from build123d import *

# Parameters (mm, degrees)
BOSS_EXTRUDE1_DEPTH = 25
FILLET1_R           = 70
FILLET2_R           = 5
CHAMFER1_SIZE       = 1
SKETCH2_R           = 2.25
CUT_EXTRUDE1_DEPTH  = 163.385344166
SKETCH5_W           = 8
SKETCH5_H           = 7
CUT_EXTRUDE2_DEPTH  = 322.199315068
CHAMFER2_SIZE       = 1


with BuildPart() as part:
    # Sketch1 → Boss-Extrude1 (new body)
    with BuildSketch(Plane(origin=(0, 0, 0), x_dir=(0, 0, -1), z_dir=(1, 0, 0))):
        Polygon((-160, 0), (160, 0), (160, -5), (100, -12), (-100, -12), (-160, -5), align=None)
    extrude(amount=BOSS_EXTRUDE1_DEPTH)

    # Fillet1
    fillet1_edges = [part.edges().sort_by_distance(p)[0] for p in [
        (12.5, -12, -100),
        (12.5, -12, 100),
    ]]
    fillet(fillet1_edges, radius=FILLET1_R)

    # Fillet2
    fillet2_edges = [part.edges().sort_by_distance(p)[0] for p in [
        (12.5, -5, -160),
        (12.5, -5, 160),
    ]]
    fillet(fillet2_edges, radius=FILLET2_R)

    # Chamfer1
    chamfer1_edges = [part.edges().sort_by_distance(p)[0] for p in [
        (25, -0.274710282, 160),
        (0, -8.522077997, -129.810760023),
        (25, -8.522077997, -129.810760023),
        (0, -12, 0),
        (0, -11.882005486, 99.99314025),
        (0, -11.882005486, -99.99314025),
        (25, -12, 0),
        (25, -11.882005486, 99.99314025),
        (25, -11.882005486, -99.99314025),
        (0, -0.274710282, -160),
        (25, -0.274710282, -160),
        (0, -8.522077997, 129.810760023),
        (0, -3.873798889, 158.73477024),
        (0, -3.873798889, -158.73477024),
        (25, -8.522077997, 129.810760023),
        (25, -3.873798889, 158.73477024),
        (25, -3.873798889, -158.73477024),
        (0, -0.274710282, 160),
    ]]
    chamfer(chamfer1_edges, length=CHAMFER1_SIZE)

    # Sketch2 → Cut-Extrude1 (cut, through all)
    with BuildSketch(Plane.XZ.offset(12)):
        with Locations(Location((12.5, 144, 0), (0, 0, 270))):
            Circle(SKETCH2_R)
        with Locations(Location((12.5, 112, 0), (0, 0, 270))):
            Circle(SKETCH2_R)
        with Locations(Location((12.5, 48, 0), (0, 0, 270))):
            Circle(SKETCH2_R)
        with Locations(Location((12.5, 80, 0), (0, 0, 270))):
            Circle(SKETCH2_R)
        with Locations(Location((12.5, -80, 0), (0, 0, 90))):
            Circle(SKETCH2_R)
        with Locations(Location((12.5, -48, 0), (0, 0, 90))):
            Circle(SKETCH2_R)
        with Locations(Location((12.5, -112, 0), (0, 0, 90))):
            Circle(SKETCH2_R)
        with Locations(Location((12.5, -144, 0), (0, 0, 90))):
            Circle(SKETCH2_R)
        with Locations(Location((12.5, 16, 0), (0, 0, 270))):
            Circle(SKETCH2_R)
        with Locations(Location((12.5, -16, 0), (0, 0, 90))):
            Circle(SKETCH2_R)
    extrude(amount=-CUT_EXTRUDE1_DEPTH, mode=Mode.SUBTRACT)

    # Sketch5 → Cut-Extrude2 (cut, through all)
    with BuildSketch(Plane.XY.offset(160)):
        with Locations((12.5, -8.5)):
            Rectangle(SKETCH5_W, SKETCH5_H)
    extrude(amount=-CUT_EXTRUDE2_DEPTH, mode=Mode.SUBTRACT)

    # Chamfer2
    # the kernel refuses this chamfer: 1 mm, written as the material it takes off along each edge
    with BuildSketch(Plane(origin=(16.5, -0.549420563, 155), x_dir=(0, -0.5507413136369002, 0.8346759883053434), z_dir=(0, 0.8346759883053434, 0.5507413136369002))) as chamfer2_piece_1_section:
        Polygon((5, CHAMFER2_SIZE), (5 - CHAMFER2_SIZE, 0), (5, 0), align=None)
    chamfer2_piece_1 = revolve(axis=Axis((16.5, -0.549420563, 155), (1, 0, 0)), revolution_arc=49.927689897, mode=Mode.PRIVATE)
    chamfer2_piece_1 = split(chamfer2_piece_1, bisect_by=Plane(origin=(16.914516826, -5, 156.211106637), z_dir=(0, -1, 0)), keep=Keep.TOP, mode=Mode.PRIVATE)
    add(chamfer2_piece_1, mode=Mode.SUBTRACT)
    with BuildSketch(Plane(origin=(8.5, -0.549420563, 155), x_dir=(0, -0.5507413136369004, 0.8346759883053431), z_dir=(0, 0.8346759883053431, 0.5507413136369004))) as chamfer2_piece_2_section:
        Polygon((5 - CHAMFER2_SIZE, 0), (5, -CHAMFER2_SIZE), (5, 0), align=None)
    chamfer2_piece_2 = revolve(axis=Axis((8.5, -0.549420563, 155), (1, 0, 0)), revolution_arc=49.927689897, mode=Mode.PRIVATE)
    chamfer2_piece_2 = split(chamfer2_piece_2, bisect_by=Plane(origin=(8.085483174, -5, 156.211106637), z_dir=(0, -1, 0)), keep=Keep.TOP, mode=Mode.PRIVATE)
    add(chamfer2_piece_2, mode=Mode.SUBTRACT)
    with BuildSketch(Plane(origin=(8.5, 58, -95.930467578), x_dir=(0, -1, 0), z_dir=(0, 0, 1))) as chamfer2_piece_3:
        Polygon((70, -CHAMFER2_SIZE), (70 - CHAMFER2_SIZE, 0), (70, 0), align=None)
    revolve(axis=Axis((8.5, 58, -95.930467578), (1, 0, 0)), revolution_arc=6.654425046, mode=Mode.SUBTRACT)
    with BuildSketch(Plane(origin=(8.5, -0.549420563, -155), x_dir=(0, -0.9932631390872432, -0.11588069956017648), z_dir=(0, -0.11588069956017648, 0.9932631390872432))) as chamfer2_piece_4_section:
        Polygon((5 - CHAMFER2_SIZE, 0), (5, -CHAMFER2_SIZE), (5, 0), align=None)
    chamfer2_piece_4 = revolve(axis=Axis((8.5, -0.549420563, -155), (1, 0, 0)), revolution_arc=49.927689897, mode=Mode.PRIVATE)
    chamfer2_piece_4 = split(chamfer2_piece_4, bisect_by=Plane(origin=(8.085483174, -5, -156.211106637), z_dir=(0, -1, 0)), keep=Keep.TOP, mode=Mode.PRIVATE)
    add(chamfer2_piece_4, mode=Mode.SUBTRACT)
    with BuildSketch(Plane(origin=(8.5, 58, 95.930467578), x_dir=(0, -0.9932631390872428, 0.11588069956017871), z_dir=(0, 0.11588069956017871, 0.9932631390872428))) as chamfer2_piece_5:
        Polygon((70 - CHAMFER2_SIZE, 0), (70, -CHAMFER2_SIZE), (70, 0), align=None)
    revolve(axis=Axis((8.5, 58, 95.930467578), (1, 0, 0)), revolution_arc=6.654425046, mode=Mode.SUBTRACT)
    with BuildSketch(Plane(origin=(16.5, 58, -95.930467578), x_dir=(0, -1, 0), z_dir=(0, 0, 1))) as chamfer2_piece_6:
        Polygon((70 - CHAMFER2_SIZE, 0), (70, CHAMFER2_SIZE), (70, 0), align=None)
    revolve(axis=Axis((16.5, 58, -95.930467578), (1, 0, 0)), revolution_arc=6.654425046, mode=Mode.SUBTRACT)
    with BuildSketch(Plane(origin=(16.5, -0.549420563, -155), x_dir=(0, -0.9932631390872432, -0.11588069956017648), z_dir=(0, -0.11588069956017648, 0.9932631390872432))) as chamfer2_piece_7_section:
        Polygon((5, CHAMFER2_SIZE), (5 - CHAMFER2_SIZE, 0), (5, 0), align=None)
    chamfer2_piece_7 = revolve(axis=Axis((16.5, -0.549420563, -155), (1, 0, 0)), revolution_arc=49.927689897, mode=Mode.PRIVATE)
    chamfer2_piece_7 = split(chamfer2_piece_7, bisect_by=Plane(origin=(16.914516826, -5, -156.211106637), z_dir=(0, -1, 0)), keep=Keep.TOP, mode=Mode.PRIVATE)
    add(chamfer2_piece_7, mode=Mode.SUBTRACT)
    with BuildSketch(Plane(origin=(16.5, 58, 95.930467578), x_dir=(0, -0.9932631390872428, 0.11588069956017871), z_dir=(0, 0.11588069956017871, 0.9932631390872428))) as chamfer2_piece_8:
        Polygon((70 - CHAMFER2_SIZE, 0), (70, CHAMFER2_SIZE), (70, 0), align=None)
    revolve(axis=Axis((16.5, 58, 95.930467578), (1, 0, 0)), revolution_arc=6.654425046, mode=Mode.SUBTRACT)
    with BuildSketch(Plane(origin=(16.5, -12, 95.930467578), x_dir=(-0.0274958766105891, 0.9996219169112968, 0), z_dir=(0, 0, -1))) as chamfer2_piece_9:
        Polygon((CHAMFER2_SIZE * 0.999621916911, CHAMFER2_SIZE * 0.0274958766106), (-CHAMFER2_SIZE * 0.0274958766106, CHAMFER2_SIZE * 0.999621916911), (0, 0), align=None)
    extrude(amount=191.860935157, mode=Mode.SUBTRACT)
    with BuildSketch(Plane(origin=(8.5, -12, 95.930467578), x_dir=(0.02749587661058392, 0.9996219169112968, 0), z_dir=(0, 0, -1))) as chamfer2_piece_10:
        Polygon((CHAMFER2_SIZE * 0.999621916911, -CHAMFER2_SIZE * 0.0274958766106), (-CHAMFER2_SIZE * 0.0274958766106, -CHAMFER2_SIZE * 0.999621916911), (0, 0), align=None)
    extrude(amount=191.860935157, mode=Mode.SUBTRACT)
    with BuildSketch(Plane(origin=(8.5, -5.515736259, 155.579403498), x_dir=(0.02749587661058567, 0.9928876030917217, -0.11583688702736752), z_dir=(0, -0.11588069956017834, -0.993263139087243))) as chamfer2_piece_11_section:
        Polygon((CHAMFER2_SIZE * 0.999621916911, -CHAMFER2_SIZE * 0.0274958766106), (-CHAMFER2_SIZE * 0.0274958766106, -CHAMFER2_SIZE * 0.999621916911), (0, 0), align=None)
    chamfer2_piece_11 = extrude(amount=51.886841384, mode=Mode.PRIVATE)
    chamfer2_piece_11 = split(chamfer2_piece_11, bisect_by=Plane(origin=(8.17503416, -5, 154.587318638), z_dir=(0, -1, 0)), keep=Keep.TOP, mode=Mode.PRIVATE)
    add(chamfer2_piece_11, mode=Mode.SUBTRACT)
    with BuildSketch(Plane(origin=(8.5, -11.528419736, -104.042116548), x_dir=(-0.9996219169112968, -0.027310640714189302, -0.0031862414166552175), z_dir=(0, 0.11588069956017857, -0.993263139087243))) as chamfer2_piece_12_section:
        Polygon((CHAMFER2_SIZE * 0.999621916911, CHAMFER2_SIZE * 0.0274958766106), (-CHAMFER2_SIZE * 0.0274958766106, CHAMFER2_SIZE * 0.999621916911), (0, 0), align=None)
    chamfer2_piece_12 = extrude(amount=51.886841384, mode=Mode.PRIVATE)
    chamfer2_piece_12 = split(chamfer2_piece_12, bisect_by=Plane(origin=(8.158054196, -5, -132.007867246), z_dir=(0, -1, 0)), keep=Keep.TOP, mode=Mode.PRIVATE)
    add(chamfer2_piece_12, mode=Mode.SUBTRACT)
    with BuildSketch(Plane(origin=(16.5, -5.515736259, -155.579403498), x_dir=(-0.027495876610589238, 0.9928876030917216, 0.11583688702736777), z_dir=(0, -0.11588069956017857, 0.993263139087243))) as chamfer2_piece_13_section:
        Polygon((CHAMFER2_SIZE * 0.999621916911, -CHAMFER2_SIZE * 0.0274958766106), (-CHAMFER2_SIZE * 0.0274958766106, -CHAMFER2_SIZE * 0.999621916911), (0, 0), align=None)
    chamfer2_piece_13 = extrude(amount=51.886841384, mode=Mode.PRIVATE)
    chamfer2_piece_13 = split(chamfer2_piece_13, bisect_by=Plane(origin=(16.82496584, -5, -154.587318638), z_dir=(0, -1, 0)), keep=Keep.TOP, mode=Mode.PRIVATE)
    add(chamfer2_piece_13, mode=Mode.SUBTRACT)
    with BuildSketch(Plane(origin=(16.5, -11.528419736, 104.042116548), x_dir=(-0.02749587661058908, 0.9928876030917217, -0.11583688702736755), z_dir=(0, 0.11588069956017834, 0.993263139087243))) as chamfer2_piece_14_section:
        Polygon((CHAMFER2_SIZE * 0.999621916911, -CHAMFER2_SIZE * 0.0274958766106), (-CHAMFER2_SIZE * 0.0274958766106, -CHAMFER2_SIZE * 0.999621916911), (0, 0), align=None)
    chamfer2_piece_14 = extrude(amount=51.886841384, mode=Mode.PRIVATE)
    chamfer2_piece_14 = split(chamfer2_piece_14, bisect_by=Plane(origin=(16.785811772, -5, 107.657614918), z_dir=(0, -1, 0)), keep=Keep.TOP, mode=Mode.PRIVATE)
    add(chamfer2_piece_14, mode=Mode.SUBTRACT)


solid = part.part
The listing builds one solid part. Answer for the finished solid, in the listing's coordinates (mm). A direction names the side the tool comes from. Coordinates: 2 decimals unless noted, no trailing zeros. Loops run counter-clockwise (first coordinate to the right, second up) from the corner with the lowest first, then second, coordinate; pieces in that order, holes last. Notation, with made-up numbers: (12, 53) -> (65, 53) arc R5 cw to (65, 61) -> close; hole circle Ø4 at (-3, -18.5). An arc over 180 degrees is marked (long way). Answer in a Markdown table with one row per item. Add a question column.
1. The part is cut by section C-C, the plane y = -8.5. Write down the section's boundary in (x, z).
2. The part is cut by section D-D, the plane z = -134. Write down the section's boundary in (x, y).
3. Flat-ended cylindrical pins translate along their axes: P1, Ø3.5, axis at x = 12.5, z = -16, coming from the +Y side; P2, Ø7, axis at x = 12.5, z = -48, coming from the +Y side; P3, Ø3, axis at x = 14.5, z = 65, coming from the -Y side; P4, Ø1.5, axis at x = 10, y = -4, coming from the +Z side. Find the tip coordinate at first contact, or state that the pin passes through.
4. The part is cut by section B-B, the plane z = 92. Write down the section's boundary in (x, y).
5. Determine the mould class of faces 3 (the flat face through (20.704, -8.564, 129.45)), 4 (the flat face through (16.99, -8.06, 129.39)), 5 (the flat face through (8.007, -7.976, 130.113)), 6 (the flat face through (0.49, -8.06, 129.39)) for opening direction X: +X half, -X half, draft (parallel to the pull), parting line (faces both ways), or undercut.
6. The part is cut by section A-A, the plane x = 4. Write down the section's boundary in (y, z).
7. For faces 1 (the cylindrical face through (4.3, -11.88, -100.05)), 2 (the flat face through (8.5, -8, 2)), determine the directions among +Z, -Z, +X, -X, +Y, -Y from which every point of the face is accessible in a straight line to the end or side of a thin tool.
8. Consider line 1 (X direction, y = -3.7, z = 80); line 2 (X direction, y = -9, z = 102); line 3 (Y direction, x = 13.5, z = 22). Determine where each line is inside the solid, lowest interval first. Write a range as [from, to].
Answer below:
| question | item | result |
|---|---|---|
| 1 | outline | (0, -121.37) -> (1, -130) -> (7.5, -130) -> (8.5, -121.37) -> (8.5, 121.37) -> (7.5, 130) -> (1, 130) -> (0, 121.37) -> close; (16.5, -121.37) -> (17.5, -130) -> (24, -130) -> (25, -121.37) -> (25, 121.37) -> (24, 130) -> (17.5, 130) -> (16.5, 121.37) -> close |
| 2 | outline | (0, -7.03) -> (1, -8.03) -> (7.5, -8.03) -> (8.5, -7.03) -> (8.5, -5) -> (16.5, -5) -> (16.5, -7.03) -> (17.5, -8.03) -> (24, -8.03) -> (25, -7.03) -> (25, 0) -> (0, 0) -> close |
| 3 | P1 | through |
| 3 | P2 | y = 0 |
| 3 | P3 | y = -5 |
| 3 | P4 | z = 159.21 |
| 4 | outline | (0, -11) -> (1, -12) -> (7.5, -12) -> (8.5, -11) -> (8.5, -5) -> (16.5, -5) -> (16.5, -11) -> (17.5, -12) -> (24, -12) -> (25, -11) -> (25, 0) -> (0, 0) -> close |
| 5 | face 3 | draft |
| 5 | face 4 | undercut |
| 5 | face 5 | undercut |
| 5 | face 6 | -X half |
| 6 | outline | (-12, -95.93) arc R70 ccw to (-11.53, -104.04) -> (-5.52, -155.58) arc R5 ccw to (-0.55, -160) -> (0, -160) -> (0, 160) -> (-0.55, 160) arc R5 ccw to (-5.52, 155.58) -> (-11.53, 104.04) arc R70 ccw to (-12, 95.93) -> close |
| 7 | face 1 | -Z, +X, -X, -Y |
| 7 | face 2 | +Z, -Z, -Y |
| 8 | line 1 | [0, 10.25], [14.75, 25] |
| 8 | line 2 | [0, 8.5], [16.5, 25] |
| 8 | line 3 | [-5, 0] |
